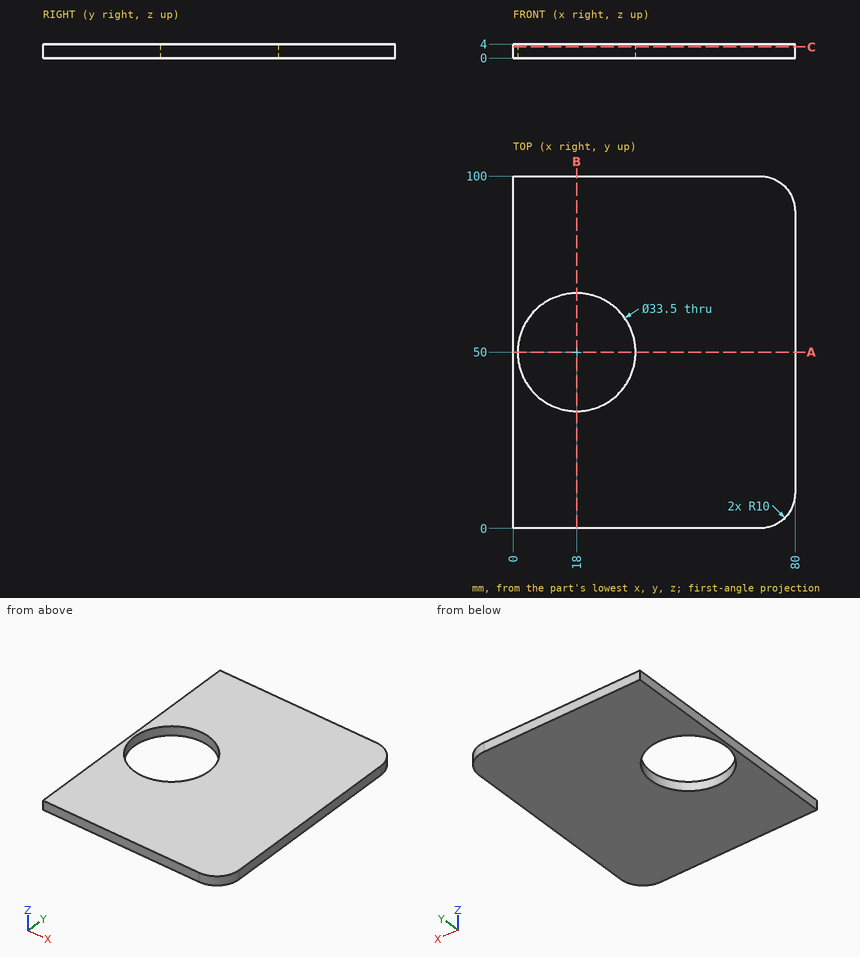
The figure shows three views and two pictorial views of one solid part (mm, origin at its lowest corner). Answer the questions. Coordinates: 2 decimals unless noted, no trailing zeros. Loops run counter-clockwise (first coordinate to the right, second up) from the corner with the lowest first, then second, coordinate; pieces in that order, holes last.
1) Find the intervals of material crossed by L1, parallel to Y at x = 18.5, z = 1.45; L2, parallel to Y at x = 28.5, z = 1.7; L3, parallel to X at y = 58.5, z = 1, in increasing order.
2) Find section B-B on x = 18. Write down the section's boundary in (y, z).
3) Find section C-C on z = 3.15. Write down the section's boundary in (x, y), then the cut area to 3 significant figures.
4) Find section A-A on y = 50. Write down the section's boundary in (x, z), then the cut area to 3 significant figures.
Values:
1. L1: y = 0 to 33.26, 66.74 to 100
1. L2: y = 0 to 36.95, 63.05 to 100
1. L3: x = 0 to 3.57, 32.43 to 80
2. outline: (0, 0) - (33.25, 0) - (33.25, 4) - (0, 4) - close; (66.75, 0) - (100, 0) - (100, 4) - (66.75, 4) - close
3. outline: (0, 0) - (70, 0) arc R10 ccw to (80, 10) - (80, 90) arc R10 ccw to (70, 100) - (0, 100) - close; hole circle Ø33.5 at (18, 50)
3. area: 7,080 mm2
4. outline: (0, 0) - (1.25, 0) - (1.25, 4) - (0, 4) - close; (34.75, 0) - (80, 0) - (80, 4) - (34.75, 4) - close
4. area: 186 mm2
